Geometry check sheet. Reference: the model listing, model coordinates, mm. Face numbers are marked on the shaded views. A direction names the side the tool comes from. Coordinates: 2 decimals unless noted, no trailing zeros. Loops run counter-clockwise (first coordinate to the right, second up) from the corner with the lowest first, then second, coordinate; pieces in that order, holes last. Notation, with made-up numbers: (7, -13.75) - (60, -13.75) arc R28 cw to (60, 13.25) - close; hole circle Ø4 at (-8, 78.5). An arc over 180 degrees is marked (long way). One line per item, written item: value.
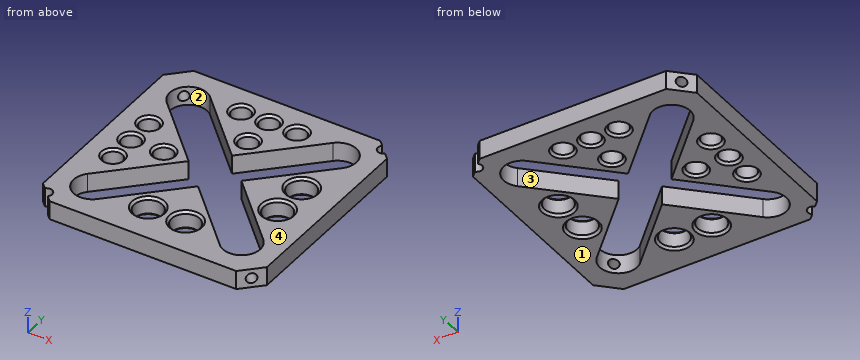
from build123d import *

# Parameters (mm, degrees)
SKETCH1_W            = 76.2
SKETCH1_H            = 76.2
EXTRUSION1_DEPTH     = 6.35
EXTRUSION2_DEPTH     = 55.254423783
MIRROR2_COPY_1_DEPTH = 55.254423783
SKETCH3_R            = 1.984375
EXTRUSION3_DEPTH     = 55.254423783
HOLE3_START          = -49.391408666
HOLE3_OUTLINE_R      = 1.7272
HOLE3_DEPTH          = 13.470384182
MIRROR4_START        = 35.921024484
MIRROR4_OUTLINE_R    = 1.7272
MIRROR4_DEPTH        = 13.470384182


with BuildPart() as part:
    # Sketch1 → Extrusion1 (new body)
    with BuildSketch(Plane.XY):
        Rectangle(SKETCH1_W, SKETCH1_H)
        with BuildLine():
            ThreePointArc((-29.890128061, -20.909871939), (-29.890128061, -29.890128061), (-20.909871939, -29.890128061))
            Line((-20.909871939, -29.890128061), (0, -8.980256121))
            Line((0, -8.980256121), (20.909871939, -29.890128061))
            ThreePointArc((20.909871939, -29.890128061), (29.890128061, -29.890128061), (29.890128061, -20.909871939))
            Line((29.890128061, -20.909871939), (8.980256121, 0))
            Line((8.980256121, 0), (29.890128061, 20.909871939))
            ThreePointArc((29.890128061, 20.909871939), (29.890128061, 29.890128061), (20.909871939, 29.890128061))
            Line((20.909871939, 29.890128061), (0, 8.980256121))
            Line((0, 8.980256121), (-20.909871939, 29.890128061))
            ThreePointArc((-20.909871939, 29.890128061), (-29.890128061, 29.890128061), (-29.890128061, 20.909871939))
            Line((-29.890128061, 20.909871939), (-8.980256121, 0))
            Line((-8.980256121, 0), (-29.890128061, -20.909871939))
        make_face(mode=Mode.SUBTRACT)
    extrude(amount=EXTRUSION1_DEPTH)

    # Sketch2 → Extrusion2 (cut, through all)
    with BuildSketch(Plane.XY.offset(6.35)):
        Polygon((-38.1, 38.1), (-38.1, 31.75), (-31.75, 38.1), align=None)
    extrusion2 = extrude(amount=-EXTRUSION2_DEPTH, mode=Mode.SUBTRACT)

    # Mirror1: Extrusion2 across plane
    add(extrusion2.mirror(Plane.ZX), mode=Mode.SUBTRACT)

    # Mirror2: Extrusion2 across plane
    add(extrusion2.mirror(Plane(origin=(0, 0, 0), x_dir=(0, 0, 1), z_dir=(1, 0, 0))), mode=Mode.SUBTRACT)

    # Mirror2 copy 1 sketch → Mirror2 copy 1 (cut, through all)
    with BuildSketch(Plane(origin=(0, 0, 6.35), x_dir=(-1, 0, 0), z_dir=(0, 0, 1))):
        Polygon((-38.1, 38.1), (-38.1, 31.75), (-31.75, 38.1), align=None)
    extrude(amount=-MIRROR2_COPY_1_DEPTH, mode=Mode.SUBTRACT)

    # Sketch3 → Extrusion3 (cut, through all)
    with BuildSketch(Plane.XY.offset(6.35)):
        with Locations((34.925, 34.925)):
            Circle(SKETCH3_R)
    extrusion3 = extrude(amount=-EXTRUSION3_DEPTH, mode=Mode.SUBTRACT)

    # Mirror3: Extrusion3 across plane
    add(extrusion3.mirror(Plane(origin=(0, 0, 6.35), x_dir=(0, 0, 1), z_dir=(0.7071067811865472, 0.7071067811865478, 0))), mode=Mode.SUBTRACT)

    # Chamfer1: read off the stored shape, not the designer's step
    # Chamfer1 outline → Chamfer1 (revolve, cut)
    with BuildSketch(Plane(origin=(-17.4498, 0, 0), x_dir=(1, 0, 0), z_dir=(0, -1, 0))):
        Polygon((0, 0), (3.96875, 0), (3.175, 0.79375), (3.175, 5.55625), (3.96875, 6.35), (0, 6.35), align=None)
    revolve(axis=Axis((-17.4498, 0, 0), (0, 0, 1)), mode=Mode.SUBTRACT)

    # Chamfer1 2 outline → Chamfer1 2 (revolve, cut)
    with BuildSketch(Plane(origin=(-28.575, -9.525, 0), x_dir=(1, 0, 0), z_dir=(0, -1, 0))):
        Polygon((0, 0), (3.96875, 0), (3.175, 0.79375), (3.175, 5.55625), (3.96875, 6.35), (0, 6.35), align=None)
    revolve(axis=Axis((-28.575, -9.525, 0), (0, 0, 1)), mode=Mode.SUBTRACT)

    # Chamfer1 3 outline → Chamfer1 3 (revolve, cut)
    with BuildSketch(Plane(origin=(-28.575, 0, 0), x_dir=(1, 0, 0), z_dir=(0, -1, 0))):
        Polygon((0, 0), (3.96875, 0), (3.175, 0.79375), (3.175, 5.55625), (3.96875, 6.35), (0, 6.35), align=None)
    revolve(axis=Axis((-28.575, 0, 0), (0, 0, 1)), mode=Mode.SUBTRACT)

    # Chamfer1 4 outline → Chamfer1 4 (revolve, cut)
    with BuildSketch(Plane(origin=(-28.575, 9.525, 0), x_dir=(1, 0, 0), z_dir=(0, -1, 0))):
        Polygon((0, 0), (3.96875, 0), (3.175, 0.79375), (3.175, 5.55625), (3.96875, 6.35), (0, 6.35), align=None)
    revolve(axis=Axis((-28.575, 9.525, 0), (0, 0, 1)), mode=Mode.SUBTRACT)

    # Chamfer1 5 outline → Chamfer1 5 (revolve, cut)
    with BuildSketch(Plane(origin=(-9.525, 28.575, 0), x_dir=(1, 0, 0), z_dir=(0, -1, 0))):
        Polygon((0, 0), (3.96875, 0), (3.175, 0.79375), (3.175, 5.55625), (3.96875, 6.35), (0, 6.35), align=None)
    revolve(axis=Axis((-9.525, 28.575, 0), (0, 0, 1)), mode=Mode.SUBTRACT)

    # Chamfer1 6 outline → Chamfer1 6 (revolve, cut)
    with BuildSketch(Plane(origin=(9.525, 28.575, 0), x_dir=(1, 0, 0), z_dir=(0, -1, 0))):
        Polygon((0, 0), (3.96875, 0), (3.175, 0.79375), (3.175, 5.55625), (3.96875, 6.35), (0, 6.35), align=None)
    revolve(axis=Axis((9.525, 28.575, 0), (0, 0, 1)), mode=Mode.SUBTRACT)

    # Chamfer1 7 outline → Chamfer1 7 (revolve, cut)
    with BuildSketch(Plane.XZ.offset(-28.575)):
        Polygon((0, 0), (3.96875, 0), (3.175, 0.79375), (3.175, 5.55625), (3.96875, 6.35), (0, 6.35), align=None)
    revolve(axis=Axis((0, 28.575, 0), (0, 0, 1)), mode=Mode.SUBTRACT)

    # Chamfer1 8 outline → Chamfer1 8 (revolve, cut)
    with BuildSketch(Plane.XZ.offset(-17.4752)):
        Polygon((0, 0), (3.96875, 0), (3.175, 0.79375), (3.175, 5.55625), (3.96875, 6.35), (0, 6.35), align=None)
    revolve(axis=Axis((0, 17.4752, 0), (0, 0, 1)), mode=Mode.SUBTRACT)

    # Hole3: read off the stored shape, not the designer's step
    # Hole3 outline → Hole3 (cut)
    with BuildSketch(Plane(origin=(0, 0, 0), x_dir=(0.7071067811865471, 0.707106781186548, 0), z_dir=(0.707106781186548, -0.707106781186547, 0)).offset(HOLE3_START)):
        with Locations((0, 3.175)):
            Circle(HOLE3_OUTLINE_R)
    extrude(amount=HOLE3_DEPTH, mode=Mode.SUBTRACT)

    # Hole3 2 outline → Hole3 2 (revolve, cut)
    with BuildSketch(Plane(origin=(-6.35, -25.4, 0), x_dir=(1, 0, 0), z_dir=(0, -1, 0))):
        Polygon((0, 0), (5.55625, 0), (4.7625, 0.79375), (4.7625, 5.55625), (5.55625, 6.35), (0, 6.35), align=None)
    revolve(axis=Axis((-6.35, -25.4, 0), (0, 0, 1)), mode=Mode.SUBTRACT)

    # Hole3 3 outline → Hole3 3 (revolve, cut)
    with BuildSketch(Plane(origin=(6.35, -25.4, 0), x_dir=(1, 0, 0), z_dir=(0, -1, 0))):
        Polygon((0, 0), (5.55625, 0), (4.7625, 0.79375), (4.7625, 5.55625), (5.55625, 6.35), (0, 6.35), align=None)
    revolve(axis=Axis((6.35, -25.4, 0), (0, 0, 1)), mode=Mode.SUBTRACT)

    # Hole3 4 outline → Hole3 4 (revolve, cut)
    with BuildSketch(Plane(origin=(25.4, -6.35, 0), x_dir=(1, 0, 0), z_dir=(0, -1, 0))):
        Polygon((0, 0), (5.55625, 0), (4.7625, 0.79375), (4.7625, 5.55625), (5.55625, 6.35), (0, 6.35), align=None)
    revolve(axis=Axis((25.4, -6.35, 0), (0, 0, 1)), mode=Mode.SUBTRACT)

    # Hole3 5 outline → Hole3 5 (revolve, cut)
    with BuildSketch(Plane(origin=(25.4, 6.35, 0), x_dir=(1, 0, 0), z_dir=(0, -1, 0))):
        Polygon((0, 0), (5.55625, 0), (4.7625, 0.79375), (4.7625, 5.55625), (5.55625, 6.35), (0, 6.35), align=None)
    revolve(axis=Axis((25.4, 6.35, 0), (0, 0, 1)), mode=Mode.SUBTRACT)

    # Mirror4: read off the stored shape, not the designer's step
    # Mirror4 outline → Mirror4 (cut)
    with BuildSketch(Plane(origin=(0, 0, 0), x_dir=(0.707106781186548, 0.707106781186547, 0), z_dir=(0.707106781186547, -0.707106781186548, 0)).offset(MIRROR4_START)):
        with Locations((0, 3.175)):
            Circle(MIRROR4_OUTLINE_R)
    extrude(amount=MIRROR4_DEPTH, mode=Mode.SUBTRACT)


solid = part.part
(1) Release check for a two-part mould opening along X. For the marked faces 1 and 2 record: pulls with the +X half, pulls with the -X half, needs draft (parallel to the pull), parting line crosses it, or undercut.
Reply:
face 1: needs draft
face 2: undercut
(2) Access from +Z, -Z, +X, -X, +Y, -Y to the whole of each face (thin tool, end or side, straight path). Record for the marked faces 3 and 4.
Reply:
face 3: +Z, -Z
face 4: +Z, +X, -X, +Y, -Y
(3) Material ranges on probe 1 along Y at (x, z) = (0, 3.7); probe 2 along X at (y, z) = (-15, 3.5); probe 3 along Y at (x, z) = (-13, 2.5), recorded low to high. Write a range as from..to.
Reply:
probe 1: -38.1..-8.98, 8.98..14.3, 20.65..25.4, 31.75..38.1
probe 2: -38.1..-23.98, -6.02..6.02, 23.98..38.1
probe 3: -38.1..-21.98, -4.02..4.02, 21.98..38.1
(4) Go/stop test with flat-tipped pins: pin 1 Ø1.5 at (x, y) = (12, 3.5) entering from -Z; pin 2 Ø11 at (x, y) = (-6.35, -25.4) entering from -Z; pin 3 Ø7.5 at (x, y) = (-17.45, 0) entering from +Z. Record where each tip stops, or that it passes through.
Reply:
pin 1: z = 0
pin 2: z = 0.06
pin 3: z = 6.13
(5) Cross-section at A-A on y = -25.4. Record the cut outline in (x, z).
Reply:
outline: (-38.1, 0) - (-31.75, 0) - (-31.75, 6.35) - (-38.1, 6.35) - close; (-16.42, 0) - (-11.91, 0) - (-11.11, 0.79) - (-11.11, 5.56) - (-11.91, 6.35) - (-16.42, 6.35) - close; (-1.59, 0.79) - (-0.79, 0) - (0.79, 0) - (1.59, 0.79) - (1.59, 5.56) - (0.79, 6.35) - (-0.79, 6.35) - (-1.59, 5.56) - close; (11.11, 0.79) - (11.91, 0) - (16.42, 0) - (16.42, 6.35) - (11.91, 6.35) - (11.11, 5.56) - close; (31.75, 0) - (38.1, 0) - (38.1, 6.35) - (31.75, 6.35) - close
